Geometry check sheet. Reference: the model listing, model coordinates, mm. Face numbers are marked on the shaded views. Give positions to 0.01 mm unless a question says otherwise; leave off trailing zeros. Loops run counter-clockwise (first coordinate to the right, second up) from the corner with the lowest first, then second, coordinate; pieces in that order, holes last. Notation, with made-up numbers: (61.5, 88) -> (115.5, 88) arc R8 ccw to (115.5, 92) -> close; hole circle Ø6 at (27, 39). An arc over 180 degrees is marked (long way). Write item = value, one per line.
```python
from build123d import *

# Parameters (mm, degrees)
SKETCH1_R           = 2.5
SKETCH1_R_2         = 4
BOSS_EXTRUDE1_DEPTH = 5


with BuildPart() as part:
    # Sketch1 → Boss-Extrude1 (new body)
    with BuildSketch(Plane.XY):
        with BuildLine():
            Line((16, 16), (-16, 16))
            ThreePointArc((-16, 16), (-21.809314436, 11.5006218), (-18.905861295, 4.750621929))
            Line((-18.905861295, 4.750621929), (-2.421551079, -4.374481726))
            ThreePointArc((-2.421551079, -4.374481726), (0, -5), (2.421551079, -4.374481726))
            Line((2.421551079, -4.374481726), (18.905861295, 4.750621929))
            ThreePointArc((18.905861295, 4.750621929), (21.809314436, 11.5006218), (16, 16))
        make_face()
        Circle(SKETCH1_R, mode=Mode.SUBTRACT)
        with Locations((-16, 10)):
            Circle(SKETCH1_R_2, mode=Mode.SUBTRACT)
        with Locations((16, 10)):
            Circle(SKETCH1_R_2, mode=Mode.SUBTRACT)
    extrude(amount=BOSS_EXTRUDE1_DEPTH)


solid = part.part
```
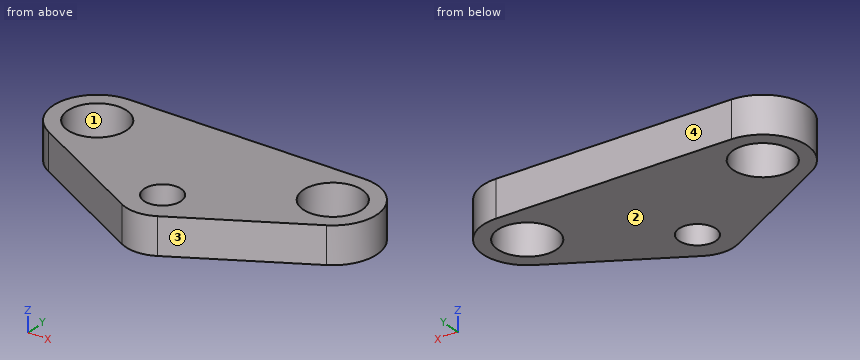
Item 1: Gauge pin test, flat ends, axial feed: pin 1 (1 mm diameter, centred on x = -6.5, z = 0.5, fed in from -Y); pin 2 (1.5 mm diameter, centred on y = 4, z = 4, fed in from -X); pin 3 (2 mm diameter, centred on y = -2.5, z = 2.5, fed in from +X). Record the tip position at first contact, or that the pin passes through.
Answer:
pin_1 = -2.39
pin_2 = -18.9
pin_3 = 7.61
Item 2: Section check A-A, the plane x = 0. Record the cut outline in (y, z).
Answer:
outline = (-5, 0) -> (-2.5, 0) -> (-2.5, 5) -> (-5, 5) -> close; (2.5, 0) -> (16, 0) -> (16, 5) -> (2.5, 5) -> close
Item 3: Section check D-D, the plane y = 0. Record the cut outline in (x, z), plus the area to 3 significant figures.
Answer:
outline = (-10.32, 0) -> (-2.5, 0) -> (-2.5, 5) -> (-10.32, 5) -> close; (2.5, 0) -> (10.32, 0) -> (10.32, 5) -> (2.5, 5) -> close
area = 78.2 mm^2
Item 4: Thickness scan on L1, parallel to X at y = 9, z = 0.9; L2, parallel to X at y = 12.75, z = 0.4; L3, parallel to X at y = -0.5, z = 1. Record the ranges inside material, lowest first. Write a range as [from, to].
Answer:
L1 = [-21.92, -19.87], [-12.13, 12.13], [19.87, 21.92]
L2 = [-21.33, -18.9], [-13.1, 13.1], [18.9, 21.33]
L3 = [-9.42, -2.45], [2.45, 9.42]
Item 5: Section check B-B, the plane y = 10. Record the cut outline in (x, z), plus the area to 3 significant figures.
Answer:
outline = (-22, 0) -> (-20, 0) -> (-20, 5) -> (-22, 5) -> close; (-12, 0) -> (12, 0) -> (12, 5) -> (-12, 5) -> close; (20, 0) -> (22, 0) -> (22, 5) -> (20, 5) -> close
area = 140 mm^2
Item 6: Draft check along Y on the marked faces 1, 2, 3 and 4. Enter one of: +Y half, -Y half, draft (parallel to the pull), parting line (faces both ways), or undercut.
Answer:
face_1 = undercut
face_2 = draft
face_3 = -Y half
face_4 = +Y half
Item 7: Section check C-C, the plane z = 1.6. Record the cut outline in (x, y).
Answer:
outline = (-18.91, 4.75) -> (-2.42, -4.37) arc R5 ccw to (2.42, -4.37) -> (18.91, 4.75) arc R6 ccw to (16, 16) -> (-16, 16) arc R6 ccw to start; hole circle Ø8 at (-16, 10); hole circle Ø5 at (0, 0); hole circle Ø8 at (16, 10)
